Input: part model. Units: mm. Frame: model coordinates. A direction names the side the tool comes from. Give positions to 0.01 mm unless a question says otherwise; leave off trailing zeros. Write each loop counter-clockwise with the first axis right and the second up, starting at its lowest first coordinate (ties: lowest second). Pieces come first, ordered by that corner, then holes. Notation, with made-up numbers: (-23, 74.5) -> (2, 74.5) arc R23 cw to (2, 99.5) -> close; hole circle Ø11 at (-34, 84). An arc over 180 degrees is marked (long way). Return JSON: item names as keys, results as strings. Group by question number.
Item 1: Pin query (flat end, axial travel): P1, Ø5, axis at x = 11, y = 6.5, coming from the +Z side; P2, Ø1.5, axis at y = -8, z = 6, coming from the +X side; P3, Ø6, axis at x = -4, y = -2, coming from the -Z side; P4, Ø4, axis at x = 5.5, z = 4, coming from the -Y side. Return the tip coordinate at first contact, or that it passes through.
Item 2: Section C-C, the plane z = 5.5. Return loops of the section in (x, y).
Item 3: Set-up query: faces 1 (the face through (15.333, -0.275, 6.725)), 2 (the face through (-1, -10, 11)). Return all of +Z, -Z, +X, -X, +Y, -Y with unobstructed straight access to the full face (end or side cutting, diameter ignored); none if empty.
Item 4: Mould query, pull axis Y, two halves, no side actions, for faces 3 (the face through (-2.38, -10.74, 5.42)), 4 (the face through (-1.269, 9.667, 5.577)), 5 (the face through (-1, -10, 0)). Classes: released by +Y, released by -Y, zero draft, split by the parting line, or undercut.
Item 5: Section A-A, the plane x = 0. Return loops of the section in (y, z), then the cut area to 3 significant figures.
Item 6: Section D-D, the plane y = 8.5. Return loops of the section in (x, z), then the cut area to 3 significant figures.
Item 7: Section B-B, the plane y = 0. Return loops of the section in (x, z), then the cut area to 3 significant figures.
Item 8: Line query: line 1 (Y direction, x = 0, z = 4.75); line 2 (Y direction, x = -7, z = 8.25); line 3 (X direction, y = -5.5, z = 1.25). Output: solid intervals per line, ascending. Write a range as [from, to].
from build123d import *

# Parameters (mm, degrees)
F0_R     = 11
F1_DEPTH = 11
F2_R     = 9.75
F3_DEPTH = 11
F5_R     = 2.116236
F6_DEPTH = 10


with BuildPart() as f1:
    # F0 (on Top) → F1 (new body)
    with BuildSketch(Plane.XY):
        Circle(F0_R)
    extrude(amount=F1_DEPTH)

    # F2 (on face) → F3 (cut)
    with BuildSketch(Plane.XY.offset(11)):
        Circle(F2_R)
    extrude(amount=-F3_DEPTH, mode=Mode.SUBTRACT)

    # F5 (on offset) → F6 (join)
    with BuildSketch(Plane.YZ.offset(10)):
        with Locations((0, 4.627058)):
            Circle(F5_R)
    extrude(amount=F6_DEPTH)


solid = f1.part
Answer below:
{
 "1": {"P1": "stops at z = 11", "P2": "stops at x = 8.27", "P3": "passes through", "P4": "stops at y = -10.43"},
 "2": {"outline": "(10.83, -1.93) -> (20, -1.93) -> (20, 1.93) -> (10.83, 1.93) arc R11 ccw (long way) to start; hole circle Ø19.5 at (0, 0)"},
 "3": {"face 1": "+X", "face 2": "+Z, +X, -X, +Y, -Y"},
 "4": {"face 3": "split by the parting line", "face 4": "undercut", "face 5": "zero draft"},
 "5": {"outline": "(-11, 0) -> (-9.75, 0) -> (-9.75, 11) -> (-11, 11) -> close; (9.75, 0) -> (11, 0) -> (11, 11) -> (9.75, 11) -> close", "area": "27.5 mm2"},
 "6": {"outline": "(-6.98, 0) -> (-4.78, 0) -> (-4.78, 11) -> (-6.98, 11) -> close; (4.78, 0) -> (6.98, 0) -> (6.98, 11) -> (4.78, 11) -> close", "area": "48.5 mm2"},
 "7": {"outline": "(-11, 0) -> (-9.75, 0) -> (-9.75, 11) -> (-11, 11) -> close; (9.75, 0) -> (11, 0) -> (11, 2.51) -> (20, 2.51) -> (20, 6.74) -> (11, 6.74) -> (11, 11) -> (9.75, 11) -> close", "area": "65.6 mm2"},
 "8": {"line 1": "y = [-11, -9.75], [9.75, 11]", "line 2": "y = [-8.49, -6.79], [6.79, 8.49]", "line 3": "x = [-9.53, -8.05], [8.05, 9.53]"}
}
